```python
from build123d import *

# Parameters (mm, degrees)
SKETCH1_R                      = 33
SKETCH1_R_2                    = 30
BOSS_EXTRUDE2_DEPTH            = 15
BOSS_EXTRUDE3_REACH            = 52.774
BOSS_EXTRUDE3_END_MAJOR_RADIUS = 23.22782186
BOSS_EXTRUDE3_END_MINOR_RADIUS = 10
SKETCH4_R                      = 25.5
SKETCH4_R_2                    = 22.55
FILLET1_R                      = 10


with BuildPart() as part:
    # Sketch1 → Boss-Extrude2 (new body)
    with BuildSketch(Plane(origin=(0, 0, 0), x_dir=(1, 0, 0), z_dir=(0, 1, 0))):
        with Locations(Location((0, 0, 0), (0, 0, 270))):
            Circle(SKETCH1_R)
        with Locations(Location((0, 0, 0), (0, 0, 270))):
            Circle(SKETCH1_R_2, mode=Mode.SUBTRACT)
    extrude(amount=BOSS_EXTRUDE2_DEPTH)

    # Sketch3 → Revolve1 (revolve)
    with BuildSketch(Plane.XY, mode=Mode.PRIVATE) as revolve1_sk:
        with BuildLine():
            Line((0, 20), (-23.550888175, 20))
            ThreePointArc((-23.550888175, 20), (-27.086422081, 19.354143467), (-30.165266452, 17.5))
            Line((-30.165266452, 17.5), (-33, 15))
            Line((-33, 15), (-30, 15))
            Line((-30, 15), (-28.792397579, 15.80876026))
            ThreePointArc((-28.792397579, 15.80876026), (-26.135776243, 17.067852492), (-23.22782186, 17.5))
            Line((-23.22782186, 17.5), (0, 17.5))
            Line((0, 17.5), (0, 20))
        make_face()
    revolve(revolve1_sk.sketch.rotate(Axis((0, 15, 0), (0, 1, 0)), 270), axis=Axis((0, 15, 0), (0, 1, 0)))

    # Boss-Extrude3: up to this torus (the profile starts inside it)
    boss_extrude3_end = Plane(origin=(0, 7.5, 0), z_dir=(0, -1, 0)) * Torus(BOSS_EXTRUDE3_END_MAJOR_RADIUS, BOSS_EXTRUDE3_END_MINOR_RADIUS, mode=Mode.PRIVATE)
    # Sketch4 → Boss-Extrude3 (add, up to the surface)
    with BuildSketch(Plane.XZ, mode=Mode.PRIVATE) as boss_extrude3_sk1:
        with Locations(Location((0, 0, 0), (0, 0, 270))):
            Circle(SKETCH4_R)
        with Locations(Location((0, 0, 0), (0, 0, 270))):
            Circle(SKETCH4_R_2, mode=Mode.SUBTRACT)
    boss_extrude3_tool1 = extrude(boss_extrude3_sk1.sketch, amount=-BOSS_EXTRUDE3_REACH, mode=Mode.PRIVATE) & boss_extrude3_end
    add(boss_extrude3_tool1.solids().sort_by_distance((0, 0, 24.778751))[0])

    # Fillet1
    # the kernel refuses this fillet: 10 mm, written as the material it takes off along each edge
    with BuildSketch(Plane(origin=(0, 15, 0), x_dir=(0, 0, -1), z_dir=(1, 0, 0))) as fillet1_piece_1:
        with BuildLine():
            CenterArc((23, -4.475597226), FILLET1_R, 0, 44.231546617)
            Line((30.165266452, 2.5), (30.308571781, 2.639511945))
            ThreePointArc((30.308571781, 2.639511945), (31.714920792, 1.4), (33.132287566, 0.15))
            Line((33.132287566, 0.15), (33.2, 0))
            Line((33.2, 0), (33.2, -4.475597226))
            Line((33.2, -4.475597226), (33, -4.475597226))
        make_face()
    revolve(axis=Axis((0, 15, 0), (0, 1, 0)), revolution_arc=180, mode=Mode.SUBTRACT)
    with BuildSketch(Plane(origin=(0, 15, 0), x_dir=(0, 0, 1), z_dir=(-1, 0, 0))) as fillet1_piece_2:
        with BuildLine():
            CenterArc((23, -4.475597226), FILLET1_R, 0, 44.231546617)
            Line((30.165266452, 2.5), (30.308571781, 2.639511945))
            ThreePointArc((30.308571781, 2.639511945), (31.714920792, 1.4), (33.132287566, 0.15))
            Line((33.132287566, 0.15), (33.2, 0))
            Line((33.2, 0), (33.2, -4.475597226))
            Line((33.2, -4.475597226), (33, -4.475597226))
        make_face()
    revolve(axis=Axis((0, 15, 0), (0, 1, 0)), revolution_arc=180, mode=Mode.SUBTRACT)


solid = part.part
```
Part model, mm, in its own coordinate system. A direction names the side the tool comes from. Give positions to 0.01 mm unless a question says otherwise; leave off trailing zeros. Write each loop counter-clockwise with the first axis right and the second up, starting at its lowest first coordinate (ties: lowest second). Pieces come first, ordered by that corner, then holes. Notation, with made-up numbers: (88.5, 8.5) -> (108.5, 8.5) arc R9 cw to (108.5, 21.5) -> close; hole circle Ø4 at (-9, 30). An arc over 180 degrees is marked (long way). Put each result on its own line as item: value. Start each with the question number.
Item 1: Cut at A-A (x = 0). List the corners of the cut face in (y, z), then the cut area to 3 significant figures.
Item 2: Wall check: L1, parallel to X at y = 11, z = 0; L2, parallel to X at y = 13.75, z = 0.5; L3, parallel to Z at x = 18, y = 8. Give the ranges that are in metal, low to high. Write a range as [from, to].
Item 3: Cut at B-B (z = 0). List the corners of the cut face in (x, y), then the cut area to 3 significant figures.
Item 4: Pull direction Z, two halves, no side cores. Call faces 1 (the face through (0, 17.5, 0)), 2 (the face through (1.32, 7.4, -29.97)), 3 (the face through (0, 20, 0)), 4 (the face through (-32.215, 5.189, -7.154)): pulls with the +Z half, pulls with the -Z half, needs draft (parallel to the pull), parting line crosses it, or undercut.
Item 5: Pin check, flat tips, straight feed: pin 1 Ø2 at (x, y) = (-14.5, 15) entering from +Z; pin 2 Ø3 at (x, y) = (20, 14) entering from +Z; pin 3 Ø8 at (x, z) = (4, 15) entering from -Y. Stop position of each tip, or through.
Item 6: Which spindle directions (+Z, -Z, +X, -X, +Y, -Y) get a long thin tool onto all of the face, cutting with end or side? Do faces 5 (the face through (-23, 0, -2)), 6 (the face through (-24.9, 8.5, 5.5)). Say none if no direction does.
Answer list:
1. outline: (0, -33) -> (10.52, -33) arc R10 ccw to (17.5, -30.17) arc R10 ccw to (20, -23.55) -> (20, 23.55) arc R10 ccw to (17.5, 30.17) arc R10 ccw to (10.52, 33) -> (0, 33) -> (0, 30) -> (15, 30) -> (15.81, 28.79) arc R10 cw to (17.24, 25.5) -> (0, 25.5) -> (0, 22.55) -> (17.48, 22.55) arc R10 ccw to (17.5, 23.23) -> (17.5, -23.23) arc R10 ccw to (17.48, -22.55) -> (0, -22.55) -> (0, -25.5) -> (17.24, -25.5) arc R10 cw to (15.81, -28.79) -> (15, -30) -> (0, -30) -> close
1. area: 347 mm2
2. L1: x = [-32.99, -30], [-25.5, -22.55], [22.55, 25.5], [30, 32.99]
2. L2: x = [-32.46, -30], [-25.5, -22.54], [22.54, 25.5], [30, 32.46]
2. L3: z = [-27.66, -24], [-18.06, -13.58], [13.58, 18.06], [24, 27.66]
3. outline: (-33, 0) -> (-30, 0) -> (-30, 15) -> (-28.79, 15.81) arc R10 cw to (-25.5, 17.24) -> (-25.5, 0) -> (-22.55, 0) -> (-22.55, 17.48) arc R10 ccw to (-23.23, 17.5) -> (23.23, 17.5) arc R10 ccw to (22.55, 17.48) -> (22.55, 0) -> (25.5, 0) -> (25.5, 17.24) arc R10 cw to (28.79, 15.81) -> (30, 15) -> (30, 0) -> (33, 0) -> (33, 10.52) arc R10 ccw to (30.17, 17.5) arc R10 ccw to (23.55, 20) -> (-23.55, 20) arc R10 ccw to (-30.17, 17.5) arc R10 ccw to (-33, 10.52) -> close
3. area: 347 mm2
4. face 1: undercut
4. face 2: undercut
4. face 3: needs draft
4. face 4: parting line crosses it
5. pin 1: stops at z = 29.17
5. pin 2: stops at z = 26.73
5. pin 3: stops at y = 17.5
6. face 5: +Z, -Z, +X, -X, -Y
6. face 6: -Y
